```python
from build123d import *

# Parameters (mm, degrees)
F0_R     = 23.01875
F0_R_2   = 2.15265
F0_R_3   = 3.96875
F0_R_4   = 11.90625
F1_DEPTH = 1.5875


with BuildPart() as f1:
    # F0 (on Top) → F1 (new body)
    with BuildSketch(Plane.XY):
        Circle(F0_R)
        with Locations((-12.347852, -12.347852)):
            Circle(F0_R_2, mode=Mode.SUBTRACT)
        with Locations((12.347852, -12.347852)):
            Circle(F0_R_3, mode=Mode.SUBTRACT)
        with Locations((-12.347852, 12.347852)):
            Circle(F0_R_3, mode=Mode.SUBTRACT)
        Circle(F0_R_4, mode=Mode.SUBTRACT)
        with Locations((12.347852, 12.347852)):
            Circle(F0_R_2, mode=Mode.SUBTRACT)
    extrude(amount=F1_DEPTH)


solid = f1.part
```
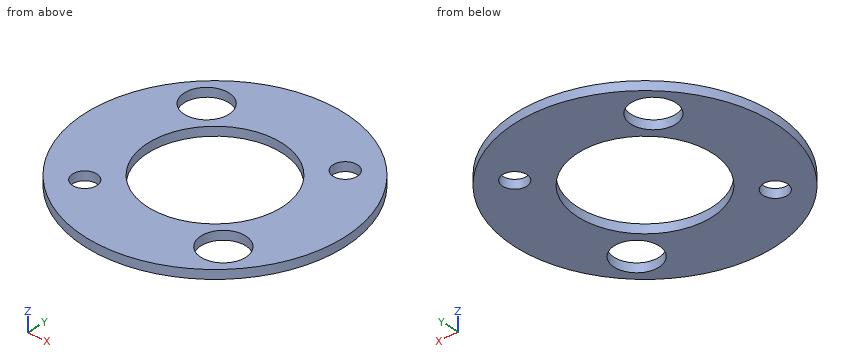
Here's how the part is built. I have some questions about the finished solid (model axes, mm). Give positions to 0.01 mm unless a question says otherwise; leave off trailing zeros. Write each loop counter-clockwise with the first axis right and the second up, starting at its lowest first coordinate (ties: lowest second). Pieces come first, ordered by that corner, then holes. Notation, with made-up numbers: (12, 67) -> (17, 67) arc R34 cw to (17, 103) -> close; hole circle Ø11 at (13.5, 55.5). An arc over 180 degrees is marked (long way). Write each question's results on one line, items separated by ' | '.
Item 1: Suppose I cut it at D-D on x = 19. Write out the boundary of the cut face in (y, z), plus the area to 3 significant figures.
Output:
outline: (-12.99, 0) -> (12.99, 0) -> (12.99, 1.59) -> (-12.99, 1.59) -> close | area: 41.3 mm^2
Item 2: Suppose I cut it at C-C on z = 0.3. Write out the boundary of the cut face in (x, y).
Output:
outline: circle Ø46.04 at (0, 0); hole circle Ø7.94 at (-12.35, 12.35); hole circle Ø4.31 at (-12.35, -12.35); hole circle Ø23.81 at (0, 0); hole circle Ø7.94 at (12.35, -12.35); hole circle Ø4.31 at (12.35, 12.35)
Item 3: If I drill on L1, parallel to X at y = -0.5, z = 1.2; L2, parallel to Y at x = 12, z = 1.45; L3, parallel to Y at x = 3, z = 1.05, over which ranges is the centre line in solid material (lowest first)?
Output:
L1: x = -23.01 to -11.9, 11.9 to 23.01 | L2: y = -19.64 to -16.3, -8.39 to 10.22, 14.47 to 19.64 | L3: y = -22.82 to -11.52, 11.52 to 22.82
Item 4: For pin 1 Ø5.5 at (x, y) = (12.35, 12.35) entering from -Z, with a flat end and sliding along its axis, tell me the tip position at first contact or that it passes through.
Output:
pin 1: stops at z = 0
Item 5: Suppose I cut it at A-A on x = 0. Write out the boundary of the cut face in (y, z), plus the area to 3 significant figures.
Output:
outline: (-23.02, 0) -> (-11.91, 0) -> (-11.91, 1.59) -> (-23.02, 1.59) -> close; (11.91, 0) -> (23.02, 0) -> (23.02, 1.59) -> (11.91, 1.59) -> close | area: 35.3 mm^2
